Source: CAD feature listing. Evaluate the final solid. Frame: model axes, mm. Face numbers are marked on the shaded views. A direction names the side the tool comes from. Give positions to 0.01 mm unless a question says otherwise; leave off trailing zeros. Order: outer loops, then holes, each group sorted by start corner. A loop starts at its lowest first (then second) coordinate and runs counter-clockwise, first axis right, second up. Notation, with made-up numbers: M 24,-36 L 80,-36 A12 ccw 80,-22 Z; hole C -10.5,-13 d2. An arc over 180 degrees is marked long. Return JSON: item names as keys, results as strings.
from build123d import *

# Parameters (mm, degrees)
SKETCH1_R           = 13.5
SKETCH1_R_2         = 2.1
BOSS_EXTRUDE1_DEPTH = 7
BOSS_EXTRUDE2_START = 7
SKETCH1_3_R         = 4
BOSS_EXTRUDE2_DEPTH = 103
CUT_EXTRUDE1_DEPTH  = 17
CHAMFER1_SIZE       = 3
FILLET3_R           = 1
CHAMFER2_SIZE       = 2


with BuildPart() as part:
    # Sketch1 → Boss-Extrude1 (new body)
    with BuildSketch(Plane(origin=(0, 0, 0), x_dir=(1, 0, 0), z_dir=(0, 1, 0))):
        with Locations(Location((0, 0, 0), (0, 0, 270))):
            Circle(SKETCH1_R)
        with Locations(Location((0, -9.5, 0), (0, 0, 270))):
            Circle(SKETCH1_R_2, mode=Mode.SUBTRACT)
        with Locations(Location((-8.227241336, 4.75, 0), (0, 0, 270))):
            Circle(SKETCH1_R_2, mode=Mode.SUBTRACT)
        with Locations(Location((8.227241336, 4.75, 0), (0, 0, 270))):
            Circle(SKETCH1_R_2, mode=Mode.SUBTRACT)
    extrude(amount=BOSS_EXTRUDE1_DEPTH)

    # Sketch1<3> → Boss-Extrude2 (add)
    with BuildSketch(Plane(origin=(0, 0, 0), x_dir=(1, 0, 0), z_dir=(0, 1, 0)).offset(BOSS_EXTRUDE2_START)):
        with Locations(Location((0, 0, 0), (0, 0, 270))):
            Circle(SKETCH1_3_R)
    extrude(amount=BOSS_EXTRUDE2_DEPTH)

    # Sketch2 → Cut-Extrude1 (cut)
    with BuildSketch(Plane(origin=(0, 110, 0), x_dir=(1, 0, 0), z_dir=(0, 1, 0))):
        with BuildLine():
            Line((-1.462019152, 2.15), (1.462019152, 2.15))
            ThreePointArc((1.462019152, 2.15), (0, -2.6), (-1.462019152, 2.15))
        make_face()
    extrude(amount=-CUT_EXTRUDE1_DEPTH, mode=Mode.SUBTRACT)

    # Chamfer1
    chamfer1_edges = [part.edges().sort_by_distance(p)[0] for p in [
        (0, 7, -4),
    ]]
    chamfer(chamfer1_edges, length=CHAMFER1_SIZE)

    # Fillet3
    fillet3_edges = [part.edges().sort_by_distance(p)[0] for p in [
        (0, 7, -13.5),
        (0, 10, -4),
        (0, 7, -7),
    ]]
    fillet(fillet3_edges, radius=FILLET3_R)

    # Chamfer2
    # the kernel refuses this chamfer: 2 mm, written as the material it adds along each edge
    with BuildSketch(Plane(origin=(0, 93, 0), x_dir=(0.003141587485879782, 0, -0.9999950652018581), z_dir=(-0.9999950652018581, 0, -0.003141587485879782))) as chamfer2_piece_1:
        Polygon((2.6, -CHAMFER2_SIZE), (2.6 - CHAMFER2_SIZE, 0), (2.6, 0), align=None)
    revolve(axis=Axis((0, 93, 0), (0, -1, 0)), revolution_arc=359.64)
    with BuildSketch(Plane(origin=(-6.605385128, 93, -2.15), x_dir=(0, 0.9996219169112968, -0.0274958766105862), z_dir=(1, 0, 0))) as chamfer2_piece_2_section:
        Polygon((CHAMFER2_SIZE * 0.999621916911, CHAMFER2_SIZE * 0.0274958766106), (-CHAMFER2_SIZE * 0.0274958766106, CHAMFER2_SIZE * 0.999621916911), (0, 0), align=None)
    chamfer2_piece_2 = extrude(amount=13.210770255, mode=Mode.PRIVATE)
    chamfer2_piece_2 = chamfer2_piece_2 & Plane(origin=(0, 93.615158387, 0), x_dir=(0.5623150583543634, 0, -0.826923076923077), z_dir=(0, 1, 0)) * Cylinder(2.6, 35, mode=Mode.PRIVATE)
    add(chamfer2_piece_2)


solid = part.part
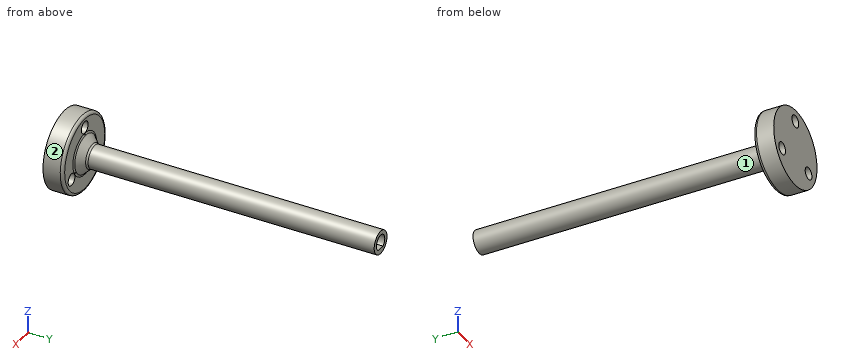
1. Section query A-A (y = 103). Return loops of the section in (x, z).
Evaluation:
{"outline": "C 0,0 d8; hole M -1.46,-2.15 L 1.46,-2.15 A2.6 ccw long Z"}
2. Section query B-B (y = 80). Return loops of the section in (x, z).
Evaluation:
{"outline": "C 0,0 d8"}
3. First-contact query: pin 1 (1.5 mm diameter, centred on x = -6.5, z = 1, fed in from +Y); pin 2 (5.5 mm diameter, centred on x = -8.23, z = -4.75, fed in from +Y); pin 3 (8 mm diameter, centred on y = 68.5, z = 7, fed in from +X). Flat tips, straight axial feed; report the tip coordinate or a pass-through.
Evaluation:
{"pin 1": "stops at y = 8.17", "pin 2": "stops at y = 7.25", "pin 3": "stops at x = 2.65"}
4. Set-up query: the marked faces 1 and 2. Return all of +Z, -Z, +X, -X, +Y, -Y with unobstructed straight access to the full face (end or side cutting, diameter ignored); none if empty.
Evaluation:
{"face 1": "+Y", "face 2": "+Y, -Y"}
5. Ray query, probe 1 along X at (y, z) = (105.5, 0); probe 2 along X at (y, z) = (2.75, -4.75); probe 3 along Z at (x, y) = (-0.25, 30). Return the intervals inside material, ascending.
Evaluation:
{"probe 1": "x = -4 to -2.6, 2.6 to 4", "probe 2": "x = -12.64 to -10.33, -6.13 to 6.13, 10.33 to 12.64", "probe 3": "z = -3.99 to 3.99"}
